from build123d import *

# Parameters (mm, degrees)
F0_R     = 9.2075
F1_DEPTH = 11.43
F2_R     = 5.08
F3_R     = 1.5875
F4_DEPTH = 25.4


with BuildPart() as f1:
    # F0 (on Front) → F1 (new body)
    with BuildSketch(Plane.XZ):
        Circle(F0_R)
    extrude(amount=F1_DEPTH)

    # F2
    f2_edges = [f1.edges().sort_by_distance(p)[0] for p in [
        (-9.2075, -11.43, 0),
        (-9.2075, 0, 0),
    ]]
    fillet(f2_edges, radius=F2_R)

    # F3 (on face) → F4 (cut)
    with BuildSketch(Plane.XZ.offset(11.43)):
        Circle(F3_R)
    extrude(amount=-F4_DEPTH, mode=Mode.SUBTRACT)


solid = f1.part
Work out the finished part from the listing and answer in its coordinate system (mm). Give positions to 0.01 mm unless a question says otherwise; leave off trailing zeros. Use a Markdown table: item, result. Add a question column.
1) For a pull along X with two mould halves and no side action, classify faces 1 (the cylindrical face through (-7.31, -5.71, -5.6)), 2 (the cylindrical face through (-0.34, -5.8, -1.55)), 3 (the flat face through (0, -11.43, -2)) as +X half, -X half, draft (parallel to the pull), parting line (faces both ways), or undercut.
2) Consider line 1 along Z through (x, y) = (0, -5.5); line 2 along Y through (x, z) = (0.25, -4.25); line 3 along Z through (x, y) = (0, -2.75). Determine where each line is inside the solid, lowest interval first.
3) Each of these flat-tipped pins is pushed along its axis until it touches: P1, Ø2, axis at x = -3.5, z = 4.5, coming from the -Y side; P2, Ø6, axis at y = -7, z = -5.5, coming from the -X side; P3, Ø4, axis at y = -9, z = -5.5, coming from the -X side. Where does it stop, or does it pass through?
Reported:
| question | item | result |
|---|---|---|
| 1 | face 1 | parting line |
| 1 | face 2 | undercut |
| 1 | face 3 | draft |
| 2 | line 1 | z = -9.21 to -1.59, 1.59 to 9.21 |
| 2 | line 2 | y = -11.43 to 0 |
| 2 | line 3 | z = -8.64 to -1.59, 1.59 to 8.64 |
| 3 | P1 | stops at y = -11.4 |
| 3 | P2 | stops at x = -8.85 |
| 3 | P3 | stops at x = -8.11 |
